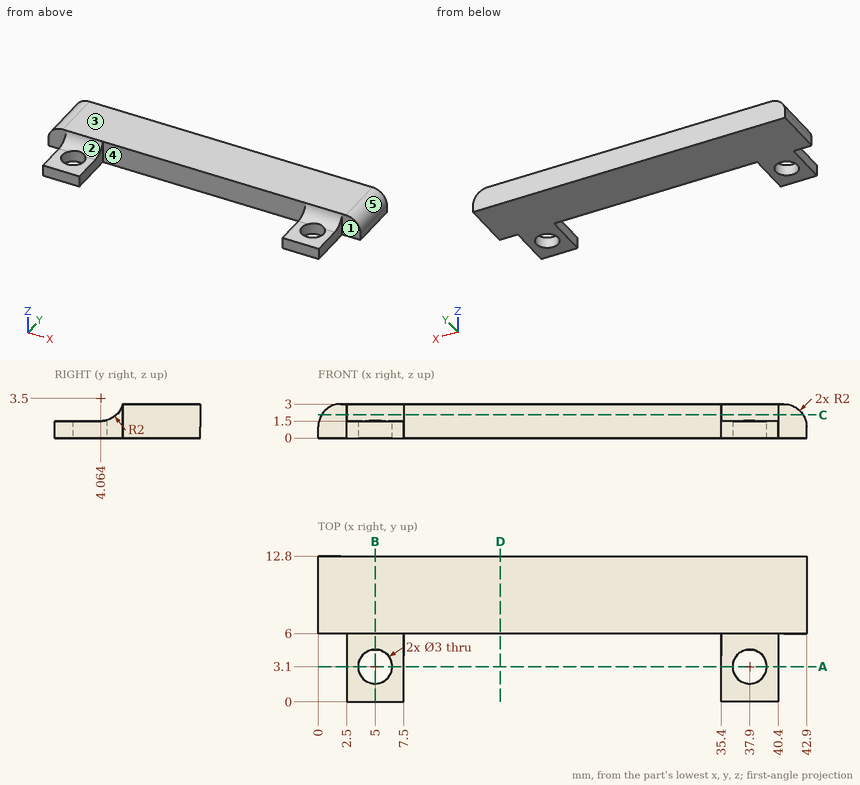
Can you work these out from the drawing? Everything is in mm from the part's minimum corner. A direction names the side the tool comes from. Coordinates: 2 decimals unless noted, no trailing zeros. Write each loop counter-clockwise with the first axis right and the second up, starting at its lowest first coordinate (ties: lowest second). Pieces come first, ordered by that corner, then holes. Notation, with made-up numbers: (32.25, 84) -> (78.25, 84) arc R6 cw to (78.25, 88) -> close; hole circle Ø9 at (70, 12.25). An arc over 180 degrees is marked (long way). Write each question's results on one line, items separated by ' | '. Start each with the question number.
Item 1: If we section it at D-D, the plane x = 16: Write out the boundary of the cut face in (y, z), and give its area (3 significant figures).
Item 2: If we section it at B-B, the plane x = 5: Write out the boundary of the cut face in (y, z).
Item 3: I'm going to push flat-ended pins straight in: P1, Ø1, axis at x = 19, z = 2, coming from the -Y side; P2, Ø4, axis at x = 37.9, y = 3.1, coming from the +Z side; P3, Ø3.5, axis at x = 4, y = 3, coming from the +Z side; P4, Ø2.5, axis at x = 5, y = 3.1, coming from the -Z side. Where does each tip first touch, or does it pass through?
Item 4: Thinking about a two-plate mould opening in X: for the marked faces 3, 4 and 5, which applies, released by +X, released by -X, zero draft, split by the parting line, or undercut?
Item 5: On a 3-axis mill with a long thin cutter (end or side, diameter ignored), from which of +Z, -Z, +X, -X, +Y, -Y can I reach the whole of each face in a straight line? I mean the marked faces 1 and 2. Say none if no direction works.
Item 6: Please list where these lines run through material, in increasing order: probe 1 along X at (y, z) = (3.1, 0.65); probe 2 along Y at (x, z) = (37.9, 1); probe 3 along Y at (x, z) = (14, 0.3).
Item 7: If we section it at C-C, the plane z = 2.05: Write out the boundary of the cut face in (x, y), and give its area (3 significant figures).
Item 8: If we section it at A-A, the plane y = 3.1: Write out the boundary of the cut face in (x, z).
Answer block:
1) outline: (6, 0) -> (12.8, 0) -> (12.8, 3) -> (6, 3) -> close | area: 20.4 mm²
2) outline: (0, 0) -> (1.6, 0) -> (1.6, 1.5) -> (0, 1.5) -> close; (4.6, 0) -> (12.8, 0) -> (12.8, 3) -> (6, 3) arc R2 cw to (4.6, 1.57) -> close
3) P1: y = 6 | P2: z = 1.79 | P3: z = 1.62 | P4: through
4) face 3: zero draft | face 4: undercut | face 5: released by +X
5) face 1: +Z, -Z, +X, -Y | face 2: +Z, +X, -X, -Y
6) probe 1: 2.5 to 3.5, 6.5 to 7.5, 35.4 to 36.4, 39.4 to 40.4 | probe 2: 0 to 1.6, 4.6 to 12.8 | probe 3: 6 to 12.8
7) outline: (0.3, 6) -> (2.5, 6) -> (2.5, 5.44) -> (7.5, 5.44) -> (7.5, 6) -> (35.4, 6) -> (35.4, 5.44) -> (40.4, 5.44) -> (40.4, 6) -> (42.6, 6) -> (42.6, 12.8) -> (0.3, 12.8) -> close | area: 293 mm²
8) outline: (2.5, 0) -> (3.5, 0) -> (3.5, 1.5) -> (2.5, 1.5) -> close; (6.5, 0) -> (7.5, 0) -> (7.5, 1.5) -> (6.5, 1.5) -> close; (35.4, 0) -> (36.4, 0) -> (36.4, 1.5) -> (35.4, 1.5) -> close; (39.4, 0) -> (40.4, 0) -> (40.4, 1.5) -> (39.4, 1.5) -> close
